Input: part model. Units: mm. Frame: model coordinates. Give positions to 0.01 mm unless a question says otherwise; leave off trailing zeros. Loops run counter-clockwise (first coordinate to the right, second up) from the corner with the lowest first, then second, coordinate; pieces in that order, holes last. Notation, with made-up numbers: M 51,-37 L 92,-37 A18 cw 92,-15 Z; hole C -38.5,-30 d2. An arc over 180 degrees is marked long. Answer as a JSON object with one key per item and string values. Group by question number.
```python
from build123d import *

# Parameters (mm, degrees)
SKETCH_1_W      = 40
SKETCH_1_H      = 80
SKETCH_1_R      = 1.6
SKETCH_1_W_2    = 4
SKETCH_1_H_2    = 14
EXTRUDE_1_DEPTH = 1
FILLET_1_R      = 3


with BuildPart() as part:
    # 草图1 → 凸台-拉伸1 (new body)
    with BuildSketch(Plane(origin=(0, 0, 0), x_dir=(1, 0, 0), z_dir=(0, 1, 0))):
        Rectangle(SKETCH_1_W, SKETCH_1_H)
        with Locations(Location((-10, -35, 0), (0, 0, 270))):
            Circle(SKETCH_1_R, mode=Mode.SUBTRACT)
        with Locations(Location((-10, -5, 0), (0, 0, 90))):
            Circle(SKETCH_1_R, mode=Mode.SUBTRACT)
        with Locations((-5, 7)):
            Rectangle(SKETCH_1_W_2, SKETCH_1_H_2, mode=Mode.SUBTRACT)
        with Locations((-15, 7)):
            Rectangle(SKETCH_1_W_2, SKETCH_1_H_2, mode=Mode.SUBTRACT)
        with Locations((5, 7)):
            Rectangle(SKETCH_1_W_2, SKETCH_1_H_2, mode=Mode.SUBTRACT)
        with Locations((15, 7)):
            Rectangle(SKETCH_1_W_2, SKETCH_1_H_2, mode=Mode.SUBTRACT)
        with Locations((-5, 29)):
            Rectangle(SKETCH_1_W_2, SKETCH_1_H_2, mode=Mode.SUBTRACT)
        with Locations((5, 29)):
            Rectangle(SKETCH_1_W_2, SKETCH_1_H_2, mode=Mode.SUBTRACT)
        with Locations((15, 29)):
            Rectangle(SKETCH_1_W_2, SKETCH_1_H_2, mode=Mode.SUBTRACT)
        with Locations((-15, 29)):
            Rectangle(SKETCH_1_W_2, SKETCH_1_H_2, mode=Mode.SUBTRACT)
    extrude(amount=EXTRUDE_1_DEPTH)

    # 圆角1
    fillet_1_edges = [part.edges().sort_by_distance(p)[0] for p in [
        (20, 0.5, 40),
        (-20, 0.5, 40),
        (-20, 0.5, -40),
        (20, 0.5, -40),
    ]]
    fillet(fillet_1_edges, radius=FILLET_1_R)


solid = part.part
```
1. Mould query, pull axis Z, two halves, no side actions, for faces 1 (the cylindrical face through (19.1, 0.51, 39.14)), 2 (the flat face through (0, 1, -1)), 3 (the cylindrical face through (-10.97, 0.49, 33.73)), 4 (the cylindrical face through (-8.44, 0.49, 5.35)). Classes: pulls with the +Z half, pulls with the -Z half, needs draft (parallel to the pull), parting line crosses it, or undercut.
2. Section A-A (z = -13). Output: boundary loops of the cut face in (x, y).
3. Section B-B (x = -4). Output: boundary loops of the cut face in (y, z), then the cut area to 3 significant figures.
4. Section C-C (z = 35). Output: boundary loops of the cut face in (x, y), then the cut area to 3 significant figures.
5. Material intervals for L1, parallel to Z at x = 16.5, y = 0.6; L2, parallel to X at y = 0.7, z = -5.5; L3, parallel to X at y = 0.85, z = 5, sorted ascending.
Geometry results:
{
 "1": {"face 1": "pulls with the +Z half", "face 2": "needs draft", "face 3": "undercut", "face 4": "undercut"},
 "2": {"outline": "M -20,0 L -17,0 L -17,1 L -20,1 Z; M -13,0 L -7,0 L -7,1 L -13,1 Z; M -3,0 L 3,0 L 3,1 L -3,1 Z; M 7,0 L 13,0 L 13,1 L 7,1 Z; M 17,0 L 20,0 L 20,1 L 17,1 Z"},
 "3": {"outline": "M 0,-40 L 1,-40 L 1,-36 L 0,-36 Z; M 0,-22 L 1,-22 L 1,-14 L 0,-14 Z; M 0,0 L 1,0 L 1,40 L 0,40 Z", "area": "52.0 mm2"},
 "4": {"outline": "M -20,0 L -11.6,0 L -11.6,1 L -20,1 Z; M -8.4,0 L 20,0 L 20,1 L -8.4,1 Z", "area": "36.8 mm2"},
 "5": {"L1": "-40 to -36, -22 to -14, 0 to 40", "L2": "-20 to -17, -13 to -7, -3 to 3, 7 to 13, 17 to 20", "L3": "-20 to -11.6, -8.4 to 20"}
}
